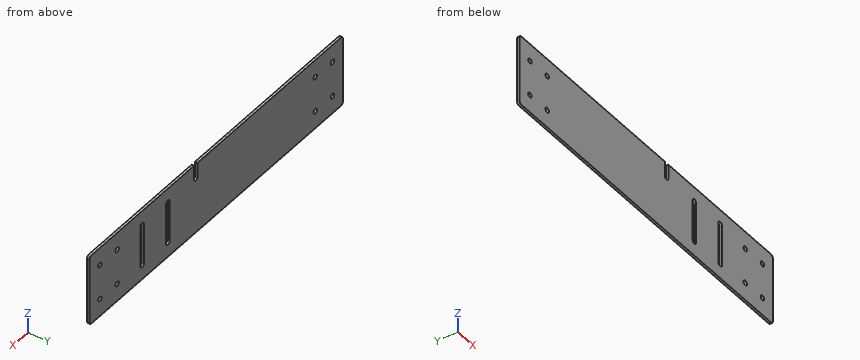
from build123d import *

# Parameters (mm, degrees)
SKETCH1_W           = 47
SKETCH1_H           = 60
SKETCH1_W_2         = 140
SKETCH1_H_2         = 140
BOSS_EXTRUDE1_DEPTH = 2
SKETCH2_R           = 2
CUT_EXTRUDE1_DEPTH  = 10
CUT_EXTRUDE3_DEPTH  = 10
FILLET1_R           = 2
SKETCH12_W          = 218.916263912
SKETCH12_H          = 42.811459275
SKETCH12_H_2        = 41.263513939
CUT_EXTRUDE4_DEPTH  = 10


with BuildPart() as part:
    # Sketch1 → Boss-Extrude1 (new body)
    with BuildSketch(Plane(origin=(0, 0, 0), x_dir=(1, 0, 0), z_dir=(0, 1, 0))):
        with Locations((-123.5, 0)):
            Rectangle(SKETCH1_W, SKETCH1_H)
        Polygon((-100, 30), (-100, -30), (-70, -70), (-70, 70), align=None)
        Rectangle(SKETCH1_W_2, SKETCH1_H_2)
        Polygon((100, 30), (100, -30), (70, -70), (70, 70), align=None)
        with Locations((123.5, 0)):
            Rectangle(SKETCH1_W, SKETCH1_H)
    extrude(amount=BOSS_EXTRUDE1_DEPTH)

    # Sketch2 → Cut-Extrude1 (cut)
    with BuildSketch(Plane(origin=(0, 2, 0), x_dir=(1, 0, 0), z_dir=(0, 1, 0))):
        with Locations(Location((-135, 15, 0), (0, 0, 270))):
            Circle(SKETCH2_R)
        with Locations(Location((-115, 15, 0), (0, 0, 270))):
            Circle(SKETCH2_R)
        with Locations(Location((-135, -15, 0), (0, 0, 270))):
            Circle(SKETCH2_R)
        with Locations(Location((-115, -15, 0), (0, 0, 270))):
            Circle(SKETCH2_R)
    cut_extrude1 = extrude(amount=-CUT_EXTRUDE1_DEPTH, mode=Mode.SUBTRACT)

    # Mirror1: Cut-Extrude1 across plane
    add(cut_extrude1.mirror(Plane(origin=(0, 0, 0), x_dir=(0, 0, 1), z_dir=(1, 0, 0))), mode=Mode.SUBTRACT)

    # Sketch11 → Cut-Extrude3 (cut)
    with BuildSketch(Plane(origin=(0, 2, 0), x_dir=(1, 0, 0), z_dir=(0, 1, 0))):
        with BuildLine():
            Line((58, -17.5), (58, 17.5))
            ThreePointArc((58, 17.5), (56, 19.5), (54, 17.5))
            Line((54, 17.5), (54, -17.5))
            ThreePointArc((54, -17.5), (56, -19.5), (58, -17.5))
        make_face()
        with BuildLine():
            Line((84, -17.5), (84, 17.5))
            ThreePointArc((84, 17.5), (86, 19.5), (88, 17.5))
            Line((88, 17.5), (88, -17.5))
            ThreePointArc((88, -17.5), (86, -19.5), (84, -17.5))
        make_face()
        with BuildLine():
            Line((21.85, -17.5), (21.85, -47.5))
            ThreePointArc((21.85, -47.5), (23.75, -49.4), (25.65, -47.5))
            Line((25.65, -47.5), (25.65, -17.5))
            ThreePointArc((25.65, -17.5), (23.75, -15.6), (21.85, -17.5))
        make_face()
    extrude(amount=-CUT_EXTRUDE3_DEPTH, mode=Mode.SUBTRACT)

    # Fillet1
    fillet1_edges = [part.edges().sort_by_distance(p)[0] for p in [
        (-147, 1, 30),
        (-147, 1, -30),
        (-100, 1, -30),
        (-70, 1, -70),
        (70, 1, -70),
        (100, 1, -30),
        (147, 1, -30),
        (147, 1, 30),
        (100, 1, 30),
        (70, 1, 70),
        (-70, 1, 70),
        (-100, 1, 30),
    ]]
    fillet(fillet1_edges, radius=FILLET1_R)

    # Sketch12 → Cut-Extrude4 (cut)
    with BuildSketch(Plane(origin=(0, 2, 0), x_dir=(1, 0, 0), z_dir=(0, 1, 0))):
        with Locations((-2.238018123, 51.405729638)):
            Rectangle(SKETCH12_W, SKETCH12_H)
        with Locations((-2.238018123, -50.63175697)):
            Rectangle(SKETCH12_W, SKETCH12_H_2)
    extrude(amount=-CUT_EXTRUDE4_DEPTH, mode=Mode.SUBTRACT)


solid = part.part
Geometry: final body of the model. Coordinates: model frame, mm. Round coordinates to 2 decimals unless told otherwise and drop trailing zeros. Loops run counter-clockwise (first coordinate to the right, second up) from the corner with the lowest first, then second, coordinate; pieces in that order, holes last. Notation, with made-up numbers: (3, 43.25) -> (16, 43.25) arc R12 ccw to (16, 55.25) -> close; hole circle Ø5 at (18.25, -28). An arc over 180 degrees is marked (long way). One line per question, with ' | ' between items. Start each with the question number.
1. Section A-A on z = 6. Output: boundary loops of the cut face in (x, y).
2. Section B-B on y = 0.5. Count the separate pieces of the cut face and the enclosed holes in it, and give its area (3 significant figures).
3. Line query: line 1 along Z through (x, y) = (-135, 1.05); line 2 along X through (y, z) = (0.6, 17.5); line 3 along X through (y, z) = (0.55, -9). Output: solid intervals per line, ascending. Write a range as [from, to].
4. Contact query for a flat-ended pin moving along its axis: pin 1 (5 mm diameter, centred on x = 135, z = 15, fed in from -Y). Output: stop coordinate, or through.
Returned:
1) outline: (-147, 0) -> (54, 0) -> (54, 2) -> (-147, 2) -> close; (58, 0) -> (84, 0) -> (84, 2) -> (58, 2) -> close; (88, 0) -> (147, 0) -> (147, 2) -> (88, 2) -> close
2) separate pieces: 1 | enclosed holes: 10 | area: 17,200 mm2
3) line 1: z = [-30, -17], [-13, 13], [17, 30] | line 2: x = [-147, 21.85], [25.65, 54], [58, 84], [88, 147] | line 3: x = [-147, 54], [58, 84], [88, 147]
4) pin 1: stops at y = 0
